Read the model definition and answer for the solid it produces. Units are mm, in the model's axes. A direction names the side the tool comes from. Coordinates: 2 decimals unless noted, no trailing zeros. Write each loop counter-clockwise with the first axis right and the second up, starting at its lowest first coordinate (ties: lowest second). Pieces come first, ordered by that corner, then holes. Notation, with made-up numbers: (80, 37.5) -> (139, 37.5) arc R22 ccw to (139, 56.5) -> close; hole circle Ø8 at (-14, -35.75). An arc over 180 degrees is marked (long way). One line per item, written item: value. Start each with the question number.
from build123d import *

# Parameters (mm, degrees)
BOSS_EXTRUDE1_DEPTH = 1
BOSS_EXTRUDE2_DEPTH = 2


with BuildPart() as part:
    # Sketch1 → Boss-Extrude1 (new body)
    with BuildSketch(Plane(origin=(0, 0, 0), x_dir=(1, 0, 0), z_dir=(0, 1, 0))):
        with BuildLine():
            Line((-13, 11), (-13, -11))
            ThreePointArc((-13, -11), (-12.414213562, -12.414213562), (-11, -13))
            Line((-11, -13), (11, -13))
            ThreePointArc((11, -13), (12.414213562, -12.414213562), (13, -11))
            Line((13, -11), (13, 11))
            ThreePointArc((13, 11), (12.414213562, 12.414213562), (11, 13))
            Line((11, 13), (-11, 13))
            ThreePointArc((-11, 13), (-12.414213562, 12.414213562), (-13, 11))
        make_face()
        with BuildLine():
            Line((-11, 12), (11, 12))
            ThreePointArc((11, 12), (11.707106781, 11.707106781), (12, 11))
            Line((12, 11), (12, -11))
            ThreePointArc((12, -11), (11.707106781, -11.707106781), (11, -12))
            Line((11, -12), (-11, -12))
            ThreePointArc((-11, -12), (-11.707106781, -11.707106781), (-12, -11))
            Line((-12, -11), (-12, 11))
            ThreePointArc((-12, 11), (-11.707106781, 11.707106781), (-11, 12))
        make_face(mode=Mode.SUBTRACT)
    extrude(amount=BOSS_EXTRUDE1_DEPTH)

    # Sketch2 → Boss-Extrude2 (add)
    with BuildSketch(Plane.XZ):
        with BuildLine():
            Line((-11, -13), (11, -13))
            ThreePointArc((11, -13), (12.414213562, -12.414213562), (13, -11))
            Line((13, -11), (13, 11))
            ThreePointArc((13, 11), (12.414213562, 12.414213562), (11, 13))
            Line((11, 13), (-11, 13))
            ThreePointArc((-11, 13), (-12.414213562, 12.414213562), (-13, 11))
            Line((-13, 11), (-13, -11))
            ThreePointArc((-13, -11), (-12.414213562, -12.414213562), (-11, -13))
        make_face()
    extrude(amount=BOSS_EXTRUDE2_DEPTH)


solid = part.part
1. For a pull along Z with two mould halves and no side action, classify faces 3 (the face through (11.715, 0.493, 11.699)), 4 (the face through (0, 0, 13)), 5 (the face through (0, 0, -13)) as +Z half, -Z half, draft (parallel to the pull), parting line (faces both ways), or undercut.
2. A cutting plane is placed at A-A on y = 0.7. Give the vertices of the cut face in (x, z), then the cut area to 3 significant figures.
3. A cutting plane is placed at C-C on z = 5. Give the vertices of the cut face in (x, y).
4. A tool of negligible diameter and unlimited length cuts with its end or side. For faces 1 (the face through (13, 0, 0)), 2 (the face through (-11.715, 0.493, -11.699)), from which of +Z, -Z, +X, -X, +Y, -Y can it reach the whole face along a straight path? Write none if from no direction.
5. A cutting plane is placed at B-B on x = -3.25. Give the vertices of the cut face in (y, z), then the cut area to 3 significant figures.
6. Find the intervals of material crossed by probe 1 along Z at (x, y) = (-5.5, 0.8); probe 2 along Y at (x, z) = (-2, -1.5), in increasing order. Write a range as from..to.
7. Given pin 1 (5 mm diameter, centred on x = -8.5, z = -3, fed in from +Y), flat-ended and moving along its own axis, determine where the tip first touches the part or whether it passes through.
Derived:
1. face 3: undercut
1. face 4: +Z half
1. face 5: -Z half
2. outline: (-13, -11) arc R2 ccw to (-11, -13) -> (11, -13) arc R2 ccw to (13, -11) -> (13, 11) arc R2 ccw to (11, 13) -> (-11, 13) arc R2 ccw to (-13, 11) -> close; hole (-12, -11) arc R1 ccw to (-11, -12) -> (11, -12) arc R1 ccw to (12, -11) -> (12, 11) arc R1 ccw to (11, 12) -> (-11, 12) arc R1 ccw to (-12, 11) -> close
2. area: 97.4 mm2
3. outline: (-13, -2) -> (13, -2) -> (13, 1) -> (12, 1) -> (12, 0) -> (-12, 0) -> (-12, 1) -> (-13, 1) -> close
4. face 1: +Z, -Z, +X, +Y, -Y
4. face 2: +Y
5. outline: (-2, -13) -> (1, -13) -> (1, -12) -> (0, -12) -> (0, 12) -> (1, 12) -> (1, 13) -> (-2, 13) -> close
5. area: 54.0 mm2
6. probe 1: z = -13..-12, 12..13
6. probe 2: y = -2..0
7. pin 1: stops at y = 0
